Part print with two shaded views. Sizes in mm from the minimum x, y, z corner. A direction names the side the tool comes from. Round coordinates to 2 decimals unless told otherwise and drop trailing zeros. Order: outer loops, then holes, each group sorted by start corner. A loop starts at its lowest first (then second) coordinate and runs counter-clockwise, first axis right, second up. Notation, with made-up numbers: (-13, -7) - (3, -7) arc R21 cw to (3, 17) - close; hole circle Ø4 at (76.25, 0.25). An arc over 180 degrees is marked (long way). Answer as CSV lines item,"result". Start each with the question number.
1. Band-saw the part on A-A on y = 9.5. List the corners of the cut face in (x, z) (3 decimals).
2. Wall check: line 1 along Y through (x, z) = (9.5, 5) (3 decimals); line 2 along Y through (x, z) = (9.5, 21.25) (3 decimals); line 3 along Z through (x, y) = (8.25, 16.25). Give the ranges that are in metal, low to high. Write a range as [from, to].
3. Band-saw the part on C-C on z = 23.5. List the corners of the cut face in (x, y) (3 decimals).
4. Pull direction X, two halves, no side cores. Call the marked faces 4, 5 and 6: released by +X, released by -X, zero draft, split by the parting line, or undercut.
5. Pin check, flat tips, straight feed: pin 1 Ø4 at (y, z) = (13, 11.5) entering from -X; pin 2 Ø6 at (y, z) = (16.5, 17.5) entering from -X; pin 3 Ø3.5 at (x, y) = (9.5, 9.5) entering from -Z; pin 4 Ø1 at (x, z) = (11, 11.5) entering from +Y. Stop position of each tip, or through.
6. Band-saw the part on D-D on x = 12.5. List the corners of the cut face in (y, z) (3 decimals).
7. 3-axis set-ups, long thin cutter, end or side, ignore diameter. For the marked faces 1, 2 and 3: which of +Z, -Z, +X, -X, +Y, -Y reach the whole face in a straight line?
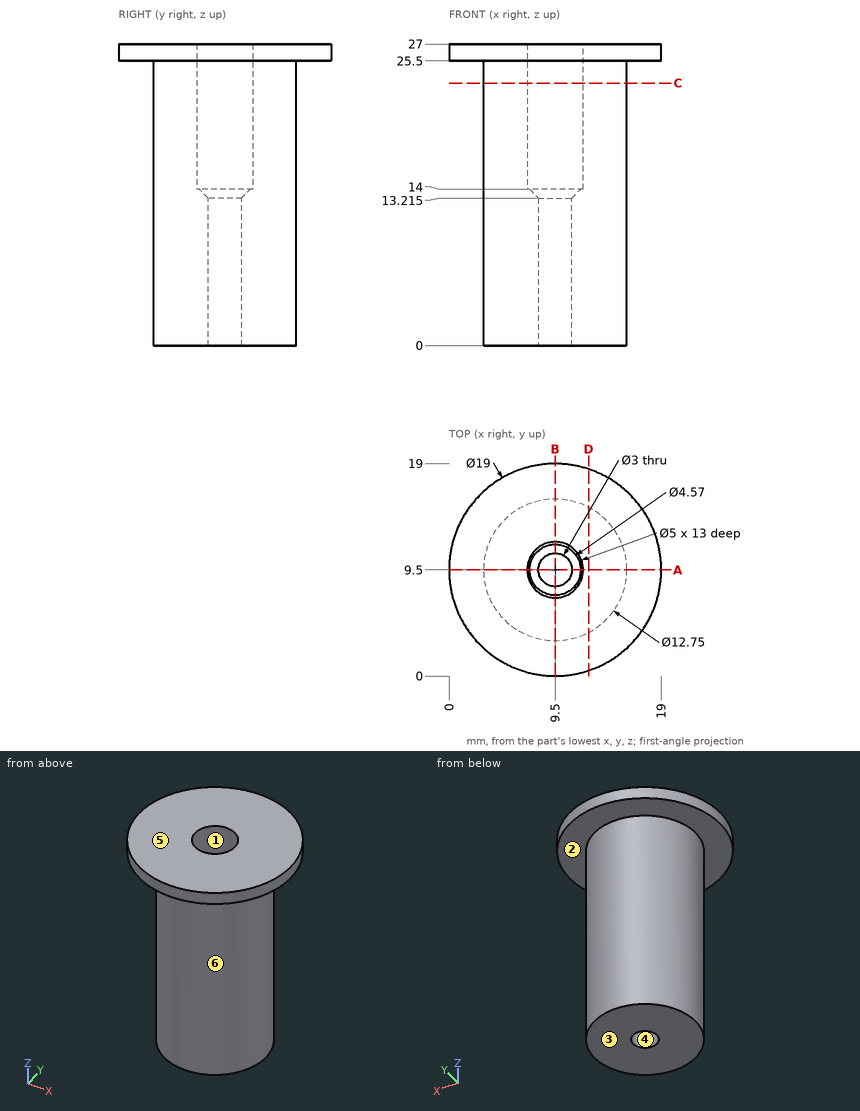
Reply:
1,outline,"(0, 25.5) - (3.125, 25.5) - (3.125, 0) - (8, 0) - (8, 13.215) - (7.215, 14) - (7, 14) - (7, 27) - (0, 27) - close; (11, 0) - (15.875, 0) - (15.875, 25.5) - (19, 25.5) - (19, 27) - (12, 27) - (12, 14) - (11.785, 14) - (11, 13.215) - close"
2,line 1,"y = [3.125, 8], [11, 15.875]"
2,line 2,"y = [3.125, 7], [12, 15.875]"
2,line 3,"z = [25.5, 27]"
3,outline,"circle Ø12.75 at (9.5, 9.5); hole circle Ø5 at (9.5, 9.5)"
4,face 4,"undercut"
4,face 5,"zero draft"
4,face 6,"split by the parting line"
5,pin 1,"stops at x = 3.3"
5,pin 2,"stops at x = 4.54"
5,pin 3,"stops at z = 0"
5,pin 4,"stops at y = 15.8"
6,outline,"(0.486, 25.5) - (3.875, 25.5) - (3.875, 0) - (15.125, 0) - (15.125, 25.5) - (18.514, 25.5) - (18.514, 27) - (0.486, 27) - close"
7,face 1,"+Z"
7,face 2,"-Z"
7,face 3,"-Z, +X, -X, +Y, -Y"
